Here's how the part is built. I have some questions about the finished solid (model axes, mm). Give positions to 0.01 mm unless a question says otherwise; leave off trailing zeros. Write each loop counter-clockwise with the first axis right and the second up, starting at its lowest first coordinate (ties: lowest second). Pieces come first, ordered by that corner, then holes. Notation, with made-up numbers: (-20.5, 46.5) - (5.5, 46.5) arc R9 cw to (5.5, 62.5) - close; hole circle Ø5 at (35, -3). An arc over 180 degrees is marked (long way). Write each question's results on one line, items separated by ' | '. Start each with the question number.
Item 1: Please list where these lines run through material, in increasing order: line 1 along Z through (x, y) = (-129, 0); line 2 along Y through (x, z) = (-134, 7.5); line 3 along Z through (x, y) = (-140.5, 8.5).
Item 2: We'd pull the mould along Y, two halves only. Please class faces 1 (the cylindrical face through (-129.58, 10.382, -19.961)), 2 (the flat face through (-130, 0, -32.5)), 3 (the flat face through (-130, -32.5, 0)): +Y half, -Y half, draft (parallel to the pull), parting line (faces both ways), or undercut.
Item 3: Suppose I cut it at A-A on y = 0. List the corners of the cut face in (x, z) for me.
Item 4: Suppose I cut it at C-C on x = -142. List the corners of the cut face in (y, z) for me, then the cut area to 3 significant figures.
```python
from build123d import *

# Parameters (mm, degrees)
F1_W     = 65
F1_H     = 65
F1_R     = 22.5
F2_DEPTH = 60


with BuildPart() as f2:
    # F1 (on offset) → F2 (new body)
    with BuildSketch(Plane.YZ.offset(-100)):
        Rectangle(F1_W, F1_H)
        Circle(F1_R, mode=Mode.SUBTRACT)
    extrude(amount=-F2_DEPTH)


solid = f2.part
```
Checked values:
1) line 1: z = -32.5 to -22.5, 22.5 to 32.5 | line 2: y = -32.5 to -21.21, 21.21 to 32.5 | line 3: z = -32.5 to -20.83, 20.83 to 32.5
2) face 1: undercut | face 2: draft | face 3: -Y half
3) outline: (-160, -32.5) - (-100, -32.5) - (-100, -22.5) - (-160, -22.5) - close; (-160, 22.5) - (-100, 22.5) - (-100, 32.5) - (-160, 32.5) - close
4) outline: (-32.5, -32.5) - (32.5, -32.5) - (32.5, 32.5) - (-32.5, 32.5) - close; hole circle Ø45 at (0, 0) | area: 2,630 mm^2
